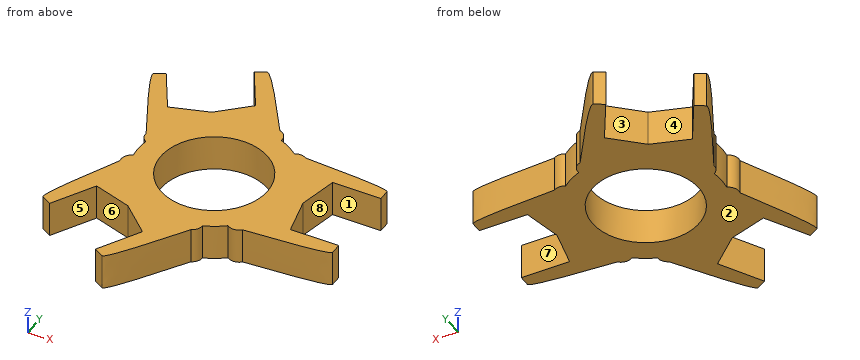
```python
from build123d import *

# Parameters (mm, degrees)
F0_R     = 9.525
F1_DEPTH = 6.35
F3_COUNT = 3
F4_R     = 9.525
F5_DEPTH = 6.35
F7_DEPTH = 6.35


with BuildPart() as f1:
    # F0 (on Top) → F1 (new body)
    with BuildSketch(Plane.XY):
        with BuildLine():
            Line((9.525, 0), (12.7, 0))
            ThreePointArc((12.7, 0), (12.1234798492, 3.7830194747), (10.4462619928, 7.2225764363))
            ThreePointArc((10.4462619928, 7.2225764363), (10.00070112, 7.0453500483), (9.525, 6.985))
            Line((9.525, 6.985), (9.525, 0))
        make_face()
        with BuildLine():
            ThreePointArc((9.525, -8.4002604126), (9.9057858228, -7.9476667791), (10.2650859452, -7.4778346155))
            ThreePointArc((10.2650859452, -7.4778346155), (9.9025309799, -7.3659812593), (9.525, -7.3281971973))
            Line((9.525, -7.3281971973), (9.525, -8.4002604126))
        make_face()
        with BuildLine():
            ThreePointArc((11.3988304843, -8.89), (11.0104940402, -8.040581393), (10.2650859452, -7.4778346155))
            ThreePointArc((10.2650859452, -7.4778346155), (9.9057858228, -7.9476667791), (9.525, -8.4002604126))
            Line((9.525, -8.4002604126), (9.525, -8.89))
            Line((9.525, -8.89), (11.3988304843, -8.89))
        make_face()
        with BuildLine():
            ThreePointArc((7.7935067776, -10.0275247248), (8.6973942383, -9.2544764013), (9.525, -8.4002604126))
            Line((9.525, -8.4002604126), (9.525, -7.3281971973))
            ThreePointArc((9.525, -7.3281971973), (7.921532049, -8.2046469895), (7.7935067776, -10.0275247248))
        make_face()
        with BuildLine():
            Line((9.525, 6.985), (9.525, 8.4002604126))
            ThreePointArc((9.525, 8.4002604126), (8.7581956911, 9.196956466), (7.9249969146, 9.9239318772))
            ThreePointArc((7.9249969146, 9.9239318772), (7.8518793788, 7.9791254823), (9.525, 6.985))
        make_face()
        with BuildLine():
            ThreePointArc((10.4462619928, 7.2225764363), (12.1234798492, 3.7830194747), (12.7, 0))
            Line((12.7, 0), (15.875, 0))
            Line((15.875, 0), (17.399, 6.9088))
            Line((17.399, 6.9088), (26.035, 6.9088))
            Line((26.035, 6.9088), (26.035, 8.89))
            Line((26.035, 8.89), (11.43, 8.89))
            ThreePointArc((11.43, 8.89), (11.1657359776, 7.922006998), (10.4462619928, 7.2225764363))
        make_face()
        with BuildLine():
            ThreePointArc((9.525, 6.985), (10.00070112, 7.0453500483), (10.4462619928, 7.2225764363))
            ThreePointArc((10.4462619928, 7.2225764363), (10.0029776208, 7.8249880969), (9.525, 8.4002604126))
            Line((9.525, 8.4002604126), (9.525, 6.985))
        make_face()
        with BuildLine():
            ThreePointArc((9.525, 8.4002604126), (10.0029776208, 7.8249880969), (10.4462619928, 7.2225764363))
            ThreePointArc((10.4462619928, 7.2225764363), (11.1657359776, 7.922006998), (11.43, 8.89))
            Line((11.43, 8.89), (9.525, 8.89))
            Line((9.525, 8.89), (9.525, 8.4002604126))
        make_face()
        with BuildLine():
            Line((9.525, -8.89), (9.525, -8.4002604126))
            ThreePointArc((9.525, -8.4002604126), (8.6973942383, -9.2544764013), (7.7935067776, -10.0275247248))
            ThreePointArc((7.7935067776, -10.0275247248), (9.9315282348, -11.0943150857), (11.43, -9.2331971973))
            ThreePointArc((11.43, -9.2331971973), (11.4221916182, -9.0608923403), (11.3988304843, -8.89))
            Line((11.3988304843, -8.89), (9.525, -8.89))
        make_face()
        with BuildLine():
            ThreePointArc((7.9249969146, 9.9239318772), (8.7581956911, 9.196956466), (9.525, 8.4002604126))
            Line((9.525, 8.4002604126), (9.525, 8.89))
            Line((9.525, 8.89), (11.43, 8.89))
            ThreePointArc((11.43, 8.89), (10.0639893887, 10.7171604852), (7.9249969146, 9.9239318772))
        make_face()
        with BuildLine():
            Line((15.875, 0), (12.7, 0))
            ThreePointArc((12.7, 0), (12.075938711, -3.9321373638), (10.2650859452, -7.4778346155))
            ThreePointArc((10.2650859452, -7.4778346155), (11.0104940402, -8.040581393), (11.3988304843, -8.89))
            Line((11.3988304843, -8.89), (26.035, -8.89))
            Line((26.035, -8.89), (26.035, -6.9088))
            Line((26.035, -6.9088), (17.399, -6.9088))
            Line((17.399, -6.9088), (15.875, 0))
        make_face()
        with BuildLine():
            ThreePointArc((10.2650859452, -7.4778346155), (12.075938711, -3.9321373638), (12.7, 0))
            Line((12.7, 0), (9.525, 0))
            Line((9.525, 0), (9.525, -7.3281971973))
            ThreePointArc((9.525, -7.3281971973), (9.9025309799, -7.3659812593), (10.2650859452, -7.4778346155))
        make_face()
        with BuildLine():
            Line((9.525, -7.3281971973), (9.525, 0))
            Line((9.525, 0), (9.525, 6.985))
            ThreePointArc((9.525, 6.985), (7.8518793788, 7.9791254823), (7.9249969146, 9.9239318772))
            ThreePointArc((7.9249969146, 9.9239318772), (-12.6997241984, 0.0836975719), (7.7935067776, -10.0275247248))
            ThreePointArc((7.7935067776, -10.0275247248), (7.921532049, -8.2046469895), (9.525, -7.3281971973))
        make_face()
        Circle(F0_R, mode=Mode.SUBTRACT)
    extrude(amount=F1_DEPTH)


with BuildPart() as f3_1:
    # F3: instance of F1
    add(f1.part.rotate(Axis((0, 0, 3.175), (0, 0, 1)), 1 * 360 / F3_COUNT))


with BuildPart() as f3_2:
    # F3: instance of F1
    add(f1.part.rotate(Axis((0, 0, 3.175), (0, 0, 1)), 2 * 360 / F3_COUNT))


with BuildPart() as f1_1:
    add(f1.part)

    add(f3_1.part)  # F5 merges F3_1

    add(f3_2.part)  # F5 merges F3_2
    # F4 (on face) → F5 (join)
    with BuildSketch(Plane.XY.offset(6.35)):
        with BuildLine():
            ThreePointArc((4.8414628101, -12.6972894296), (11.1904325012, -7.7094190078), (13.589, 0))
            ThreePointArc((13.589, 0), (-0.9329227135, 13.5569383052), (-13.4609045126, -1.8614431777))
            ThreePointArc((-13.4609045126, -1.8614431777), (-13.0283174584, -1.7464719499), (-12.5808445376, -1.7356124916))
            ThreePointArc((-12.5808445376, -1.7356124916), (6.4223463228, 10.9564349909), (4.6318786538, -11.8252145916))
            ThreePointArc((4.6318786538, -11.8252145916), (4.7887256176, -12.2487417548), (4.8414628101, -12.6972894296))
        make_face()
        with BuildLine():
            ThreePointArc((-12.5808445376, -1.7356124916), (-13.0283174584, -1.7464719499), (-13.4609045126, -1.8614431777))
            ThreePointArc((-13.4609045126, -1.8614431777), (-6.9229751419, -11.6933030486), (4.8414628101, -12.6972894296))
            ThreePointArc((4.8414628101, -12.6972894296), (4.7887256176, -12.2487417548), (4.6318786538, -11.8252145916))
            ThreePointArc((4.6318786538, -11.8252145916), (6.4223463228, 10.9564349909), (-12.5808445376, -1.7356124916))
        make_face()
        Circle(F4_R, mode=Mode.SUBTRACT)
    extrude(amount=-F5_DEPTH)

    # F6 (on face) → F7 (join)
    with BuildSketch(Plane.XY.offset(6.35)):
        with BuildLine():
            add(Edge.make_bspline(
                [(10.6367632499, 10.4369348649), (18.6027915748, 10.0299773304), (25.9883071623, 9.6007507753), (26.035, 8.89)],
                knots=[0.0462368838, 0.0462368838, 0.0462368838, 0.0462368838, 0.584525149, 0.584525149, 0.584525149, 0.584525149], degree=3))
            ThreePointArc((10.6367632499, 10.4369348649), (11.2201303771, 9.7592283961), (11.43, 8.89))
            Line((11.43, 8.89), (26.035, 8.89))
        make_face()
        with BuildLine():
            ThreePointArc((1.9995505975, 14.3166767728), (2.8133537712, 14.7235401011), (3.7230379132, 14.7065655527))
            add(Edge.make_bspline(
                [(3.7230379132, 14.7065655527), (-0.6351401044, 21.3148502374), (-4.6685883244, 27.3160665919), (-5.3185341604, 26.9919713875)],
                knots=[0.0562643988, 0.0562643988, 0.0562643988, 0.0562643988, 0.5862434824, 0.5862434824, 0.5862434824, 0.5862434824], degree=3))
            Line((-5.3185341604, 26.9919713875), (1.9995505975, 14.3166767728))
        make_face()
        with BuildLine():
            add(Edge.make_bspline(
                [(10.8747404145, -10.5775281884), (18.7767718356, -10.1073776533), (25.9907017622, -9.6149172072), (26.035, -8.89)],
                knots=[0.0562643988, 0.0562643988, 0.0562643988, 0.0562643988, 0.5862434824, 0.5862434824, 0.5862434824, 0.5862434824], degree=3))
            Line((26.035, -8.89), (11.3988304843, -8.89))
            ThreePointArc((11.3988304843, -8.89), (11.3442828756, -9.7982058862), (10.8747404145, -10.5775281884))
        make_face()
        with BuildLine():
            Line((-13.4139658396, 5.4536703653), (-20.7164658396, 18.1019713875))
            add(Edge.make_bspline(
                [(-14.3570323556, 3.993239756), (-17.987610955, 11.0955014199), (-21.3086476479, 17.7061588163), (-20.7164658396, 18.1019713875)],
                knots=[0.0462368838, 0.0462368838, 0.0462368838, 0.0462368838, 0.584525149, 0.584525149, 0.584525149, 0.584525149], degree=3))
            ThreePointArc((-14.3570323556, 3.993239756), (-14.0618049009, 4.8373037423), (-13.4139658396, 5.4536703653))
        make_face()
        with BuildLine():
            add(Edge.make_bspline(
                [(3.7202691057, -14.4301746209), (-0.6151806199, -21.1254787503), (-4.6796595144, -27.3069095915), (-5.3185341604, -26.9919713875)],
                knots=[0.0462368838, 0.0462368838, 0.0462368838, 0.0462368838, 0.584525149, 0.584525149, 0.584525149, 0.584525149], degree=3))
            ThreePointArc((3.7202691057, -14.4301746209), (2.8416745238, -14.5965321384), (1.9839658396, -14.3436703653))
            Line((1.9839658396, -14.3436703653), (-5.3185341604, -26.9919713875))
        make_face()
        with BuildLine():
            ThreePointArc((-13.3983810818, -5.4266767728), (-14.1576366468, -4.9253342149), (-14.5977783276, -4.1290373643))
            add(Edge.make_bspline(
                [(-14.5977783276, -4.1290373643), (-18.1416317312, -11.207472584), (-21.3221134379, -17.7011493846), (-20.7164658396, -18.1019713875)],
                knots=[0.0562643988, 0.0562643988, 0.0562643988, 0.0562643988, 0.5862434824, 0.5862434824, 0.5862434824, 0.5862434824], degree=3))
            Line((-20.7164658396, -18.1019713875), (-13.3983810818, -5.4266767728))
        make_face()
    extrude(amount=-F7_DEPTH)


solid = f1_1.part
```
The listing builds one solid part. Answer for the finished solid, in the listing's coordinates (mm). Face numbers are marked on the shaded views. A direction names the side the tool comes from. Round coordinates to 2 decimals unless told otherwise and drop trailing zeros. Loops run counter-clockwise (first coordinate to the right, second up) from the corner with the lowest first, then second, coordinate; pieces in that order, holes last. Notation, with made-up numbers: (32.25, 63.25) - (74.25, 63.25) arc R6 ccw to (74.25, 74.25) - close; hole circle Ø5 at (85, 23.25). An arc over 180 degrees is marked (long way). Return JSON: item names as keys, results as strings. Group by question number.
1. Each of these flat-tipped pins is pushed along its axis until it touches: P1, Ø1.5, axis at x = 4, z = 3, coming from the -Y side; P2, Ø6, axis at x = 20, y = 2, coming from the -Z side; P3, Ø1.9, axis at x = 24, z = 2.5, coming from the -Y side. Where does it stop, or does it pass through?
2. Consider probe 1 along Y at (x, z) = (-4.5, 4); probe 2 along X at (y, z) = (7, 1.75) (3 decimals); probe 3 along X at (y, z) = (-14, 3.25). Determine where each line is inside the solid, lowest interval first.
3. The part is cut by section A-A on y = -1. Determine the outline of the cut face in (x, z), then the cut area to 3 significant figures.
4. Which of the six approach directions +Z, -Z, +X, -X, +Y, -Y give full straight-line access (tool end or side, diameter ignored) to the marked faces 1, 2, 3, 4 and 5?
5. The mould has two halves that part along X. Classify the marked faces 6, 7 and 8: pulls with the +X half, pulls with the -X half, needs draft (parallel to the pull), parting line crosses it, or undercut.
Resolved:
{
 "1": {"P1": "stops at y = -15.16", "P2": "passes through", "P3": "stops at y = -9.65"},
 "2": {"probe 1": "y = -26.4 to -21.61, -16.89 to -8.39, 8.39 to 16.89, 21.61 to 26.42", "probe 2": "x = -15.888 to -6.46, 6.46 to 26.035", "probe 3": "x = -19.38 to -16.06, -7.66 to 4.32"},
 "3": {"outline": "(-13.55, 0) - (-9.47, 0) - (-9.47, 6.35) - (-13.55, 6.35) - close; (9.47, 0) - (16.1, 0) - (16.1, 6.35) - (9.47, 6.35) - close", "area": "68.0 mm²"},
 "4": {"face 1": "+Z, -Z, +X", "face 2": "-Z, +X, -X, +Y, -Y", "face 3": "+Z, -Z", "face 4": "+Z, -Z, +Y", "face 5": "+Z, -Z, -Y"},
 "5": {"face 6": "undercut", "face 7": "needs draft", "face 8": "pulls with the +X half"}
}
